Source: three-view drawing plus pictorial views. Frame: mm from the lowest corner of the part. A direction names the side the tool comes from. Give positions to 0.01 mm unless a question says otherwise; leave off trailing zeros. Loops run counter-clockwise (first coordinate to the right, second up) from the corner with the lowest first, then second, coordinate; pieces in that order, holes last. Notation, with made-up numbers: M -13,58.5 L 23,58.5 A18 ccw 23,64.5 Z; hole C -20.75,-35.5 d7. An arc over 180 degrees is marked long. Answer as a JSON object with one key per item and string values. Group by question number.
1) Access query for the marked faces 1 and 2. Directions: +Z, -Z, +X, -X, +Y, -Y. A direction counts if a zero-diameter tool reaches every point of the face in a straight line with its end or side. Return the directions, or none.
2) First-contact query: P1, Ø0.6, axis at y = 23.5, z = 1.5, coming from the +X side. Flat tip, straight axial feed; report the tip coordinate or a pass-through.
3) Draft query along Y for the marked faces 3, 4 and 5. Return one class per face: +Y half, -Y half, draft (parallel to the pull), parting line (faces both ways), or undercut.
4) Section query A-A on z = 1. Return loops of the section in (x, y).
5) Section query B-B on y = 25. Return loops of the section in (x, z), plus the area to 3 significant figures.
6) Ray query, L1, parallel to Y at x = 5, z = 0.95; L2, parallel to X at y = 16, z = 1.15; L3, parallel to Y at x = 6, z = 1.6. Return the intervals inside material, ascending.
7) Section query C-C on x = 5. Return loops of the section in (y, z), plus the area to 3 significant figures.
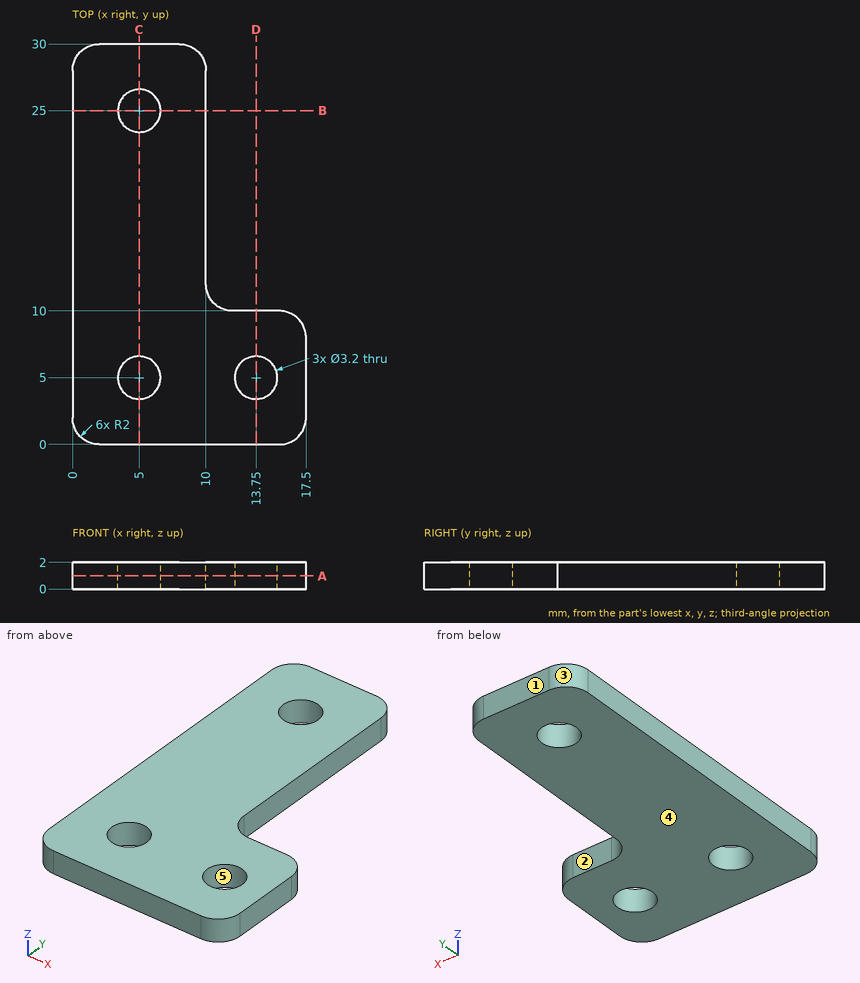
Output:
{
 "1": {"face 1": "+Z, -Z, +X, -X, +Y", "face 2": "+Z, -Z, +X, +Y"},
 "2": {"P1": "stops at x = 10"},
 "3": {"face 3": "+Y half", "face 4": "draft", "face 5": "undercut"},
 "4": {"outline": "M 0,2 A2 ccw 2,0 L 15.5,0 A2 ccw 17.5,2 L 17.5,8 A2 ccw 15.5,10 L 12,10 A2 cw 10,12 L 10,28 A2 ccw 8,30 L 2,30 A2 ccw 0,28 Z; hole C 5,5 d3.2; hole C 5,25 d3.2; hole C 13.75,5 d3.2"},
 "5": {"outline": "M 0,0 L 3.4,0 L 3.4,2 L 0,2 Z; M 6.6,0 L 10,0 L 10,2 L 6.6,2 Z", "area": "13.6 mm^2"},
 "6": {"L1": "y = 0 to 3.4, 6.6 to 23.4, 26.6 to 30", "L2": "x = 0 to 10", "L3": "y = 0 to 3.75, 6.25 to 23.75, 26.25 to 30"},
 "7": {"outline": "M 0,0 L 3.4,0 L 3.4,2 L 0,2 Z; M 6.6,0 L 23.4,0 L 23.4,2 L 6.6,2 Z; M 26.6,0 L 30,0 L 30,2 L 26.6,2 Z", "area": "47.2 mm^2"}
}
